Geometry check sheet. Reference: drawing and pictorial views, mm from the part's lowest x, y, z. Coordinates: 2 decimals unless noted, no trailing zeros. Loops run counter-clockwise (first coordinate to the right, second up) from the corner with the lowest first, then second, coordinate; pieces in that order, holes last. Notation, with made-up numbers: (-32.5, 21) -> (7.5, 21) arc R15 cw to (7.5, 30) -> close; hole circle Ø11 at (-29.75, -21). An arc over 180 degrees is marked (long way). Use one line per item in the form item = value.
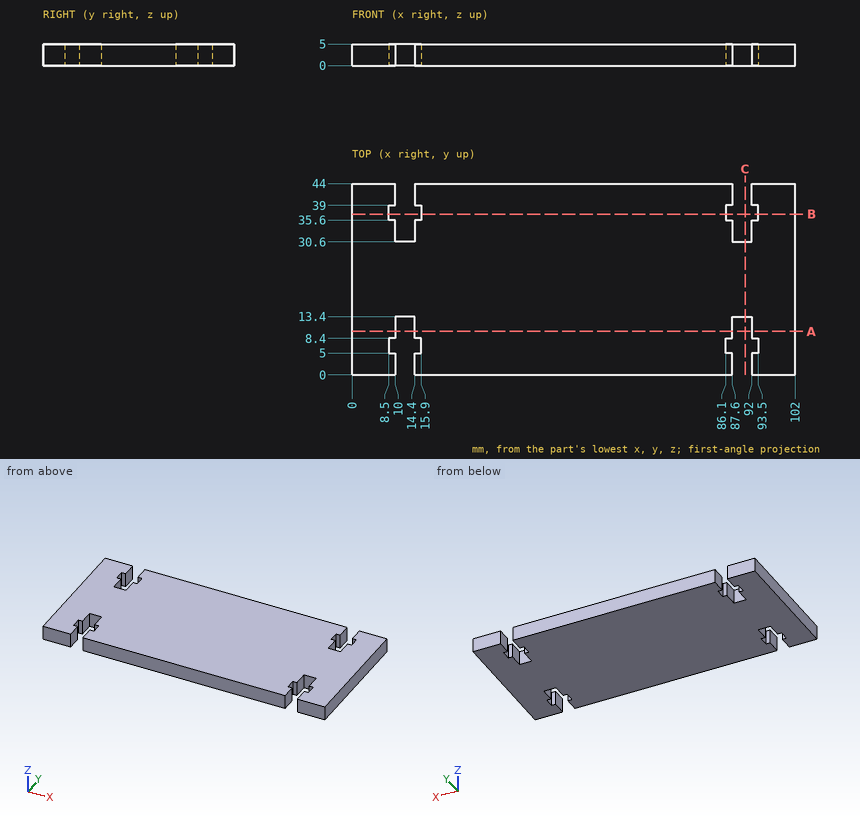
(1) Section check A-A, the plane y = 10. Record the boundary of the cut face in (x, z).
Established:
outline = (0, 0) -> (10, 0) -> (10, 5) -> (0, 5) -> close; (14.4, 0) -> (87.6, 0) -> (87.6, 5) -> (14.4, 5) -> close; (92, 0) -> (102, 0) -> (102, 5) -> (92, 5) -> close
(2) Section check C-C, the plane x = 90.5. Record the boundary of the cut face in (y, z).
Established:
outline = (13.4, 0) -> (30.6, 0) -> (30.6, 5) -> (13.4, 5) -> close
(3) Go/stop test with a flat-tipped pin: P1, Ø3, axis at y = 13, z = 1, coming from the -X side. Record where the tip stops, or that it passes through.
Established:
P1 = 0
(4) Section check B-B, the plane y = 37. Record the boundary of the cut face in (x, z).
Established:
outline = (0, 0) -> (8.5, 0) -> (8.5, 5) -> (0, 5) -> close; (15.9, 0) -> (86.1, 0) -> (86.1, 5) -> (15.9, 5) -> close; (93.5, 0) -> (102, 0) -> (102, 5) -> (93.5, 5) -> close
(5) Scan lines: line 1 along X through (y, z) = (6, 3.45); line 2 along X through (y, z) = (40, 1.7); line 3 along Y through (x, z) = (9.5, 2.3). Record each from-to range of solid material in increasing order.
Established:
line_1 = 0 to 8.5, 15.9 to 86.1, 93.5 to 102
line_2 = 0 to 10, 14.4 to 87.6, 92 to 102
line_3 = 0 to 5, 8.4 to 35.6, 39 to 44
